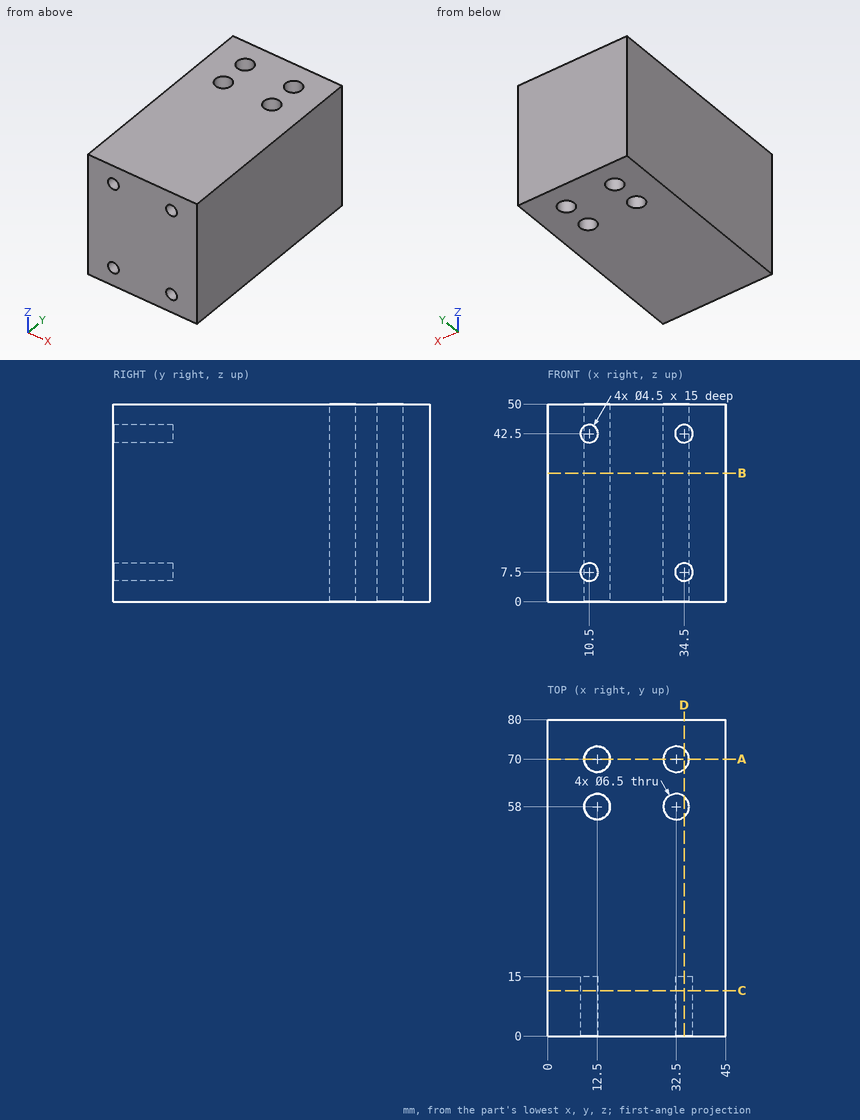
For this review, use the dimensioned drawing (mm, ordinates from the lowest corner) and the shaded views. Round coordinates to 2 decimals unless told otherwise and drop trailing zeros. Write each loop counter-clockwise with the first axis right and the second up, starting at its lowest first coordinate (ties: lowest second). Pieces come first, ordered by that corner, then holes. Notation, with made-up numbers: (-2.75, 39.25) - (34.25, 39.25) arc R24 ccw to (34.25, 66.25) - close; hole circle Ø6 at (-18, -4). An arc over 180 degrees is marked (long way). Use a Markdown table: item, result.
Q1. Clearance check with a flat-ended pin moving along its axis: pin 1 (2.5 mm diameter, centred on x = 34.5, z = 42.5, fed in from -Y). State where the tip first meets the part, or that it passes through.
Derived:
| item | result |
|---|---|
| pin 1 | stops at y = 15 |
Q2. We need section B-B (z = 32.5). Give the boundary of the cut face in (x, y), plus the area to 3 significant figures.
Derived:
| item | result |
|---|---|
| outline | (0, 0) - (45, 0) - (45, 80) - (0, 80) - close; hole circle Ø6.5 at (12.5, 58); hole circle Ø6.5 at (12.5, 70); hole circle Ø6.5 at (32.5, 58); hole circle Ø6.5 at (32.5, 70) |
| area | 3,470 mm2 |
Q3. Wall thickness on line 1 along Z through (x, y) = (34.5, 10); line 2 along Y through (x, z) = (29.5, 22.5); line 3 along Y through (x, z) = (12, 23): over which ranges is each line inside the solid? List them lowest first.
Derived:
| item | result |
|---|---|
| line 1 | z = 0 to 5.25, 9.75 to 40.25, 44.75 to 50 |
| line 2 | y = 0 to 56.75, 59.25 to 68.75, 71.25 to 80 |
| line 3 | y = 0 to 54.79, 61.21 to 66.79, 73.21 to 80 |
Q4. We need section D-D (x = 34.5). Give the boundary of the cut face in (y, z).
Derived:
| item | result |
|---|---|
| outline | (0, 0) - (55.44, 0) - (55.44, 50) - (0, 50) - (0, 44.75) - (15, 44.75) - (15, 40.25) - (0, 40.25) - (0, 9.75) - (15, 9.75) - (15, 5.25) - (0, 5.25) - close; (60.56, 0) - (67.44, 0) - (67.44, 50) - (60.56, 50) - close; (72.56, 0) - (80, 0) - (80, 50) - (72.56, 50) - close |
Q5. We need section A-A (y = 70). Give the boundary of the cut face in (x, z), plus the area to 3 significant figures.
Derived:
| item | result |
|---|---|
| outline | (0, 0) - (9.25, 0) - (9.25, 50) - (0, 50) - close; (15.75, 0) - (29.25, 0) - (29.25, 50) - (15.75, 50) - close; (35.75, 0) - (45, 0) - (45, 50) - (35.75, 50) - close |
| area | 1,600 mm2 |
Q6. We need section C-C (y = 11.5). Give the boundary of the cut face in (x, z), plus the area to 3 significant figures.
Derived:
| item | result |
|---|---|
| outline | (0, 0) - (45, 0) - (45, 50) - (0, 50) - close; hole circle Ø4.5 at (10.5, 7.5); hole circle Ø4.5 at (10.5, 42.5); hole circle Ø4.5 at (34.5, 7.5); hole circle Ø4.5 at (34.5, 42.5) |
| area | 2,190 mm2 |
